```python
from build123d import *

# Parameters (mm, degrees)
SKETCH1_R               = 27
SKETCH1_R_2             = 1.375
SKETCH1_R_3             = 20
BOSS_EXTRUDE1_DEPTH     = 10
SKETCH3_R               = 20
SKETCH3_R_2             = 1.375
BOSS_EXTRUDE2_DEPTH     = 2
BOSS_EXTRUDE3_DEPTH     = 6
CUT_EXTRUDE1_REACH      = 44.996
CUT_EXTRUDE1_END_RADIUS = 27
SKETCH4_W               = 3.5
SKETCH4_H               = 9.337272122
SKETCH6_W               = 25
SKETCH6_H               = 15.32
BOSS_EXTRUDE4_DEPTH     = 2.5
SKETCH7_R               = 1.625
BOSS_EXTRUDE5_DEPTH     = 2.5
FILLET2_R               = 10
FILLET3_R               = 1


with BuildPart() as part:
    # Sketch1 → Boss-Extrude1 (new body)
    with BuildSketch(Plane.XY):
        Circle(SKETCH1_R)
        with Locations((0, 23.5)):
            Circle(SKETCH1_R_2, mode=Mode.SUBTRACT)
        with Locations((23.5, 0)):
            Circle(SKETCH1_R_2, mode=Mode.SUBTRACT)
        with Locations((0, -23.5)):
            Circle(SKETCH1_R_2, mode=Mode.SUBTRACT)
        with Locations((-23.5, 0)):
            Circle(SKETCH1_R_2, mode=Mode.SUBTRACT)
        Circle(SKETCH1_R_3, mode=Mode.SUBTRACT)
    extrude(amount=BOSS_EXTRUDE1_DEPTH)

    # Sketch3 → Boss-Extrude2 (add)
    with BuildSketch(Plane.XY):
        Circle(SKETCH3_R)
        with Locations((-7, 0)):
            Circle(SKETCH3_R_2, mode=Mode.SUBTRACT)
        with Locations((7, 0)):
            Circle(SKETCH3_R_2, mode=Mode.SUBTRACT)
    extrude(amount=BOSS_EXTRUDE2_DEPTH)

    # Sketch5 → Boss-Extrude3 (add)
    with BuildSketch(Plane.XY.offset(10)):
        Polygon((-12.5, 23.932195888), (-4.251935746, 23.932195888), (0, 26.25446737), (4.267780323, 23.932195888), (12.5, 23.932195888), (12.5, 31.932195888), (-12.5, 31.932195888), align=None)
    extrude(amount=-BOSS_EXTRUDE3_DEPTH)

    # Cut-Extrude1: up to this cylinder (the profile starts inside it)
    cut_extrude1_end = Plane(origin=(0, 0, 8.168636), z_dir=(0, 0, -1)) * Cylinder(CUT_EXTRUDE1_END_RADIUS, 144.992, mode=Mode.PRIVATE)
    # Sketch4 → Cut-Extrude1 (cut, up to the surface)
    with BuildSketch(Plane(origin=(0, 0, 0), x_dir=(1, 0, 0), z_dir=(0, 1, 0)), mode=Mode.PRIVATE) as cut_extrude1_sk1:
        with Locations((-7.75, -8.168636061)):
            Rectangle(SKETCH4_W, SKETCH4_H)
    cut_extrude1_tool1 = extrude(cut_extrude1_sk1.sketch, amount=-CUT_EXTRUDE1_REACH, mode=Mode.PRIVATE) & cut_extrude1_end
    add(cut_extrude1_tool1.solids().sort_by_distance((-7.75, 0, 8.168636))[0], mode=Mode.SUBTRACT)

    # Sketch6 → Boss-Extrude4 (add)
    with BuildSketch(Plane(origin=(0, 31.932195888, 0), x_dir=(1, 0, 0), z_dir=(0, 1, 0))):
        with Locations((0, -2.34)):
            Rectangle(SKETCH6_W, SKETCH6_H)
    boss_extrude4 = extrude(amount=-BOSS_EXTRUDE4_DEPTH)

    # Sketch7 → Boss-Extrude5 (add)
    with BuildSketch(Plane(origin=(0, 31.932195888, 0), x_dir=(1, 0, 0), z_dir=(0, 1, 0))):
        with BuildLine():
            Line((-36.25, -9.68), (-28.75, -9.68))
            Line((-28.75, -9.68), (0, -9.68))
            Line((0, -9.68), (0, 5.32))
            Line((0, 5.32), (-32.25, 5.32))
            ThreePointArc((-32.25, 5.32), (-35.078427125, 4.148427125), (-36.25, 1.32))
            Line((-36.25, 1.32), (-36.25, -2.18))
            Line((-36.25, -2.18), (-36.25, -9.68))
        make_face()
        with Locations(Location((-28.75, -2.18, 0), (0, 0, 270))):
            Circle(SKETCH7_R, mode=Mode.SUBTRACT)
    boss_extrude5 = extrude(amount=-BOSS_EXTRUDE5_DEPTH)

    # Fillet2
    # the kernel refuses this fillet: 10 mm, written as the material it adds along each edge
    with BuildSketch(Plane(origin=(-12.5, 29.432195888, 9.68), x_dir=(-1, 0, 0), z_dir=(0, 1, 0))) as fillet2_piece_1:
        with BuildLine():
            CenterArc((2.509501943, 10), FILLET2_R, 255.466253099, 14.533746901)
            Line((0, 0.32), (-0.050190039, 0.1264))
            ThreePointArc((-0.050190039, 0.1264), (-0.2, 0.16), (-0.2, 0))
            Line((-0.2, 0), (0, -0.2))
            Line((0, -0.2), (2.509501943, -0.2))
            Line((2.509501943, -0.2), (2.509501943, 0))
        make_face()
    extrude(amount=2.5)

    # Mirror1: Boss-Extrude4, Boss-Extrude5 across plane
    add(boss_extrude4.mirror(Plane(origin=(0, 0, 0), x_dir=(0, 0, 1), z_dir=(1, 0, 0))))
    add(boss_extrude5.mirror(Plane(origin=(0, 0, 0), x_dir=(0, 0, 1), z_dir=(1, 0, 0))))

    # Fillet3
    # the kernel refuses this fillet: 1 mm, written as the material it adds along each edge
    with BuildSketch(Plane(origin=(-12.5, 29.432195888, 4), x_dir=(0, -1, 0), z_dir=(0, 0, 1))) as fillet3_piece_1_section:
        with BuildLine():
            CenterArc((FILLET3_R, -FILLET3_R), FILLET3_R, 90, 90)
            Line((0, -FILLET3_R), (0, 0))
            Line((0, 0), (FILLET3_R, 0))
        make_face()
    fillet3_piece_1 = extrude(amount=6, mode=Mode.PRIVATE)
    fillet3_piece_1 = fillet3_piece_1 - Plane(origin=(-15.009501943, 29.204760134, 19.68), x_dir=(-1, 0, 0), z_dir=(0, -1, 0)) * Cylinder(10, 16, mode=Mode.PRIVATE)
    add(fillet3_piece_1)
    with BuildSketch(Plane(origin=(12.5, 29.432195888, 9.68), x_dir=(0, -1, 0), z_dir=(0, 0, -1))) as fillet3_piece_2:
        with BuildLine():
            CenterArc((FILLET3_R, -FILLET3_R), FILLET3_R, 90, 90)
            Line((0, -FILLET3_R), (0, 0))
            Line((0, 0), (FILLET3_R, 0))
        make_face()
    extrude(amount=5.68)
    with BuildSketch(Plane(origin=(12.5, 29.432195888, 4), x_dir=(0, -1, 0), z_dir=(-1, 0, 0))) as fillet3_piece_3:
        with BuildLine():
            CenterArc((FILLET3_R, -FILLET3_R), FILLET3_R, 90, 90)
            Line((0, -FILLET3_R), (0, 0))
            Line((0, 0), (FILLET3_R, 0))
        make_face()
    extrude(amount=25)
    with BuildSketch(Plane(origin=(-12.5, 29.432195888, 1.5), x_dir=(0, -1, 0), z_dir=(0, 0, 1))) as fillet3_piece_4a_section:
        with BuildLine():
            CenterArc((FILLET3_R, -FILLET3_R), FILLET3_R, 90, 90)
            Line((0, -FILLET3_R), (0, 0))
            Line((0, 0), (FILLET3_R, 0))
        make_face()
    fillet3_piece_4a = extrude(amount=8.5, mode=Mode.PRIVATE)
    fillet3_piece_4a = split(fillet3_piece_4a, bisect_by=Plane(origin=(-12.726395114, 29.205800773, 4), z_dir=(0, 0, -1)), keep=Keep.TOP, mode=Mode.PRIVATE)
    with BuildSketch(Plane(origin=(12.5, 29.432195888, 4), x_dir=(0, -1, 0), z_dir=(-1, 0, 0))) as fillet3_piece_4b_section:
        with BuildLine():
            CenterArc((FILLET3_R, -FILLET3_R), FILLET3_R, 90, 90)
            Line((0, -FILLET3_R), (0, 0))
            Line((0, 0), (FILLET3_R, 0))
        make_face()
    fillet3_piece_4b = extrude(amount=27.5, mode=Mode.PRIVATE)
    fillet3_piece_4b = split(fillet3_piece_4b, bisect_by=Plane(origin=(-12.5, 29.205800773, 3.773604886), z_dir=(-1, 0, 0)), keep=Keep.TOP, mode=Mode.PRIVATE)
    fillet3_piece_4 = fillet3_piece_4a & fillet3_piece_4b
    add(fillet3_piece_4)
    with BuildSketch(Plane(origin=(12.5, 29.432195888, 9.68), x_dir=(0, -1, 0), z_dir=(0, 0, -1))) as fillet3_piece_5a_section:
        with BuildLine():
            CenterArc((FILLET3_R, -FILLET3_R), FILLET3_R, 90, 90)
            Line((0, -FILLET3_R), (0, 0))
            Line((0, 0), (FILLET3_R, 0))
        make_face()
    fillet3_piece_5a = extrude(amount=8.18, mode=Mode.PRIVATE)
    fillet3_piece_5a = split(fillet3_piece_5a, bisect_by=Plane(origin=(12.726395114, 29.205800773, 4), z_dir=(0, 0, -1)), keep=Keep.TOP, mode=Mode.PRIVATE)
    with BuildSketch(Plane(origin=(15, 29.432195888, 4), x_dir=(0, -1, 0), z_dir=(-1, 0, 0))) as fillet3_piece_5b_section:
        with BuildLine():
            CenterArc((FILLET3_R, -FILLET3_R), FILLET3_R, 90, 90)
            Line((0, -FILLET3_R), (0, 0))
            Line((0, 0), (FILLET3_R, 0))
        make_face()
    fillet3_piece_5b = extrude(amount=27.5, mode=Mode.PRIVATE)
    fillet3_piece_5b = split(fillet3_piece_5b, bisect_by=Plane(origin=(12.5, 29.205800773, 3.773604886), z_dir=(1, 0, 0)), keep=Keep.TOP, mode=Mode.PRIVATE)
    fillet3_piece_5 = fillet3_piece_5a & fillet3_piece_5b
    add(fillet3_piece_5)


solid = part.part
```
Source: CAD feature listing. Evaluate the final solid. Frame: model axes, mm. A direction names the side the tool comes from. Give positions to 0.01 mm unless a question says otherwise; leave off trailing zeros. Order: outer loops, then holes, each group sorted by start corner. A loop starts at its lowest first (then second) coordinate and runs counter-clockwise, first axis right, second up. Notation, with made-up numbers: (-21, 16) -> (34, 16) arc R36 cw to (34, 51) -> close; hole circle Ø7 at (68, 31). An arc over 180 degrees is marked (long way). Use a Markdown table: item, result.
Q1. Material intervals for line 1 (Y direction, x = 7, z = 1.3) (3 decimals); line 2 (Y direction, x = -16, z = 8); line 3 (Y direction, x = -30, z = -1.75), sorted ascending. Write a range as [from, to].
A:
| item | result |
|---|---|
| line 1 | [-26.077, -1.375], [1.375, 26.077], [29.432, 31.932] |
| line 2 | [-21.75, -12], [12, 21.75], [29.43, 31.93] |
| line 3 | [29.43, 31.93] |
Q2. Pull-direction query (Y, two-part tool) for faces 1 (the face through (1, 31.932, 2)), 2 (the face through (-8.374, 0.06, 0.986)), 3 (the face through (22.126, 0.06, 4.93)), 4 (the face through (27.14, 30.7, 1.97)); classes: +Y half, -Y half, draft (parallel to the pull), parting line (faces both ways), or undercut.
A:
| item | result |
|---|---|
| face 1 | +Y half |
| face 2 | undercut |
| face 3 | undercut |
| face 4 | draft |
Q3. Access query for faces 5 (the face through (0, 0, 0)), 6 (the face through (-0.2, 27.2, 4)), 7 (the face through (24, 31, 9.68)), 8 (the face through (-26, 31, 9.68)). Directions: +Z, -Z, +X, -X, +Y, -Y. A direction counts if a zero-diameter tool reaches every point of the face in a straight line with its end or side. Return the directions, or none.
A:
| item | result |
|---|---|
| face 5 | -Z, +X, -X, -Y |
| face 6 | -Z |
| face 7 | +Z, +X, +Y |
| face 8 | +Z, -X, +Y |
Q4. Section C-C (x = 23.5). Return the cut outline in (y, z) (3 decimals).
A:
| item | result |
|---|---|
| outline | (-13.295, 0) -> (-1.375, 0) -> (-1.375, 10) -> (-13.295, 10) -> close; (1.375, 0) -> (13.295, 0) -> (13.295, 10) -> (1.375, 10) -> close; (29.432, -5.32) -> (31.932, -5.32) -> (31.932, 9.68) -> (29.432, 9.68) -> close |
Q5. Section A-A (x = -28.75). Return the cut outline in (y, z) (3 decimals), and give its area (3 significant figures).
A:
| item | result |
|---|---|
| outline | (29.432, -5.32) -> (31.932, -5.32) -> (31.932, 0.555) -> (29.432, 0.555) -> close; (29.432, 3.805) -> (31.932, 3.805) -> (31.932, 9.68) -> (29.432, 9.68) -> close |
| area | 29.4 mm^2 |
Q6. Section D-D (x = 16). Return the cut outline in (y, z).
A:
| item | result |
|---|---|
| outline | (-21.75, 0) -> (21.75, 0) -> (21.75, 10) -> (12, 10) -> (12, 2) -> (-12, 2) -> (-12, 10) -> (-21.75, 10) -> close; (29.43, -5.32) -> (31.93, -5.32) -> (31.93, 9.68) -> (29.43, 9.68) -> close |
Q7. First-contact query: P1, Ø4.5, axis at x = -7, y = 0, coming from the +Z side; P2, Ø0.8, axis at x = -24.5, y = 30.5, coming from the +Z side; P3, Ø1.6, axis at x = 0, y = 23.5, coming from the -Z side; P4, Ø7.5, axis at x = 11, z = 1.5, coming from the -Y side. Flat tips, straight axial feed; report the tip coordinate or a pass-through.
A:
| item | result |
|---|---|
| P1 | z = 2 |
| P2 | z = 9.68 |
| P3 | through |
| P4 | y = -26.01 |
Q8. Section B-B (y = 0). Return the cut outline in (x, z) (3 decimals).
A:
| item | result |
|---|---|
| outline | (-27, 0) -> (-24.875, 0) -> (-24.875, 10) -> (-27, 10) -> close; (-22.125, 0) -> (-8.375, 0) -> (-8.375, 2) -> (-20, 2) -> (-20, 10) -> (-22.125, 10) -> close; (-5.625, 0) -> (5.625, 0) -> (5.625, 2) -> (-5.625, 2) -> close; (8.375, 0) -> (22.125, 0) -> (22.125, 10) -> (20, 10) -> (20, 2) -> (8.375, 2) -> close; (24.875, 0) -> (27, 0) -> (27, 10) -> (24.875, 10) -> close |
